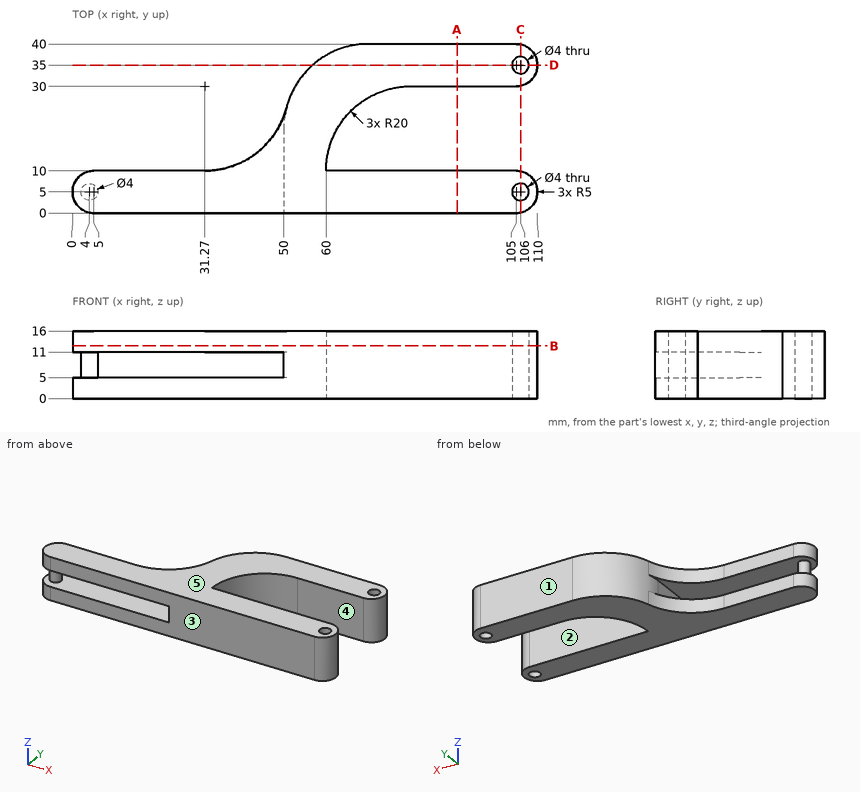
Design review of the part shown in the three views and the two pictorial views. Dimensions are in mm from the part's minimum x, y and z. A direction names the side the tool comes from. Give positions to 0.01 mm unless a question says otherwise; leave off trailing zeros. Loops run counter-clockwise (first coordinate to the right, second up) from the corner with the lowest first, then second, coordinate; pieces in that order, holes last. Notation, with made-up numbers: M 12,11.5 L 18,11.5 A16 cw 18,18.5 Z; hole C 64,61.25 d4. An arc over 180 degrees is marked long. Answer as a JSON object with one key per item and string values.
Item 1: We need section C-C (x = 106). State the section outline as (y, z) points.
Output values:
{"outline": "M 0.1,0 L 3,0 L 3,16 L 0.1,16 Z; M 7,0 L 9.9,0 L 9.9,16 L 7,16 Z; M 30.1,0 L 33,0 L 33,16 L 30.1,16 Z; M 37,0 L 39.9,0 L 39.9,16 L 37,16 Z"}
Item 2: Mouldability with a two-part tool opening along Y and no side actions: class the marked faces 1, 2 and 3 as pulls with the +Y half, pulls with the -Y half, needs draft (parallel to the pull), parting line crosses it, or undercut.
Output values:
{"face 1": "pulls with the +Y half", "face 2": "undercut", "face 3": "pulls with the -Y half"}
Item 3: Machinability: for the marked faces 4 and 5, which of the approach directions +Z, -Z, +X, -X, +Y, -Y give a long, thin tool a straight path to every point of the face, cutting with its end or side? Answer none if there is none.
Output values:
{"face 4": "+Z, -Z, +X", "face 5": "+Z, +X, -X, +Y, -Y"}
Item 4: We need section D-D (y = 35). State the section outline as (x, z) points, and give its area (3 significant figures).
Output values:
{"outline": "M 56.77,0 L 104,0 L 104,16 L 56.77,16 Z; M 108,0 L 110,0 L 110,16 L 108,16 Z", "area": "788 mm2"}
Item 5: For P1, Ø2, axis at x = 91.5, y = 27.5, coming from the -Z side; P2, Ø3, axis at y = 5.5, z = 9, coming from the -X side; P3, Ø1.5, axis at x = 16.5, z = 1.5, coming from the +Y side; P4, Ø4, axis at y = 20, z = 13.5, coming from the +X side, all flat-tipped, find the tip position at first contact; note any pin that passes through.
Output values:
{"P1": "passes through", "P2": "stops at x = 2", "P3": "stops at y = 10", "P4": "stops at x = 64"}
Item 6: Wall thickness on line 1 along Y through (x, z) = (106, 9); line 2 along Y through (x, z) = (99.5, 15); line 3 along Z through (x, y) = (29, 7): over which ranges is each line inside the solid? List them lowest first.
Output values:
{"line 1": "y = 0.1 to 3, 7 to 9.9, 30.1 to 33, 37 to 39.9", "line 2": "y = 0 to 10, 30 to 40", "line 3": "z = 0 to 5, 11 to 16"}
Item 7: We need section A-A (x = 91). State the section outline as (y, z) points.
Output values:
{"outline": "M 0,0 L 10,0 L 10,16 L 0,16 Z; M 30,0 L 40,0 L 40,16 L 30,16 Z"}
Item 8: We need section B-B (z = 12.5). Count the separate pieces of the cut face and the enclosed holes in it, and give its area (3 significant figures).
Output values:
{"separate pieces": "1", "enclosed holes": "2", "area": "1,910 mm2"}
